from build123d import *

# Parameters (mm, degrees)
SKETCH1_W             = 25.4
SKETCH1_H             = 25.4
SKETCH1_W_2           = 19.05
SKETCH1_H_2           = 19.05
BOSS_EXTRUDE1_DEPTH   = 279.4
SKETCH3_W             = 2.4892
SKETCH3_H             = 25.4
SKETCH3_AT_POINT_2_W  = 2.4892
SKETCH3_AT_POINT_2_H  = 25.4
LPATTERN1_START       = -12.7
LPATTERN1_OUTLINE_R   = 2.4892
LPATTERN1_DEPTH       = 25.4
LPATTERN1_2_OUTLINE_R = 2.4892
LPATTERN1_2_DEPTH     = 25.4


# Read off the part's stored shape, not the designer's step: LPattern1
with BuildPart() as part:
    # Sketch1 → Boss-Extrude1 (new, symmetric)
    with BuildSketch(Plane(origin=(0, 0, 0), x_dir=(0, 0, -1), z_dir=(1, 0, 0))):
        Rectangle(SKETCH1_W, SKETCH1_H)
        Rectangle(SKETCH1_W_2, SKETCH1_H_2, mode=Mode.SUBTRACT)
    extrude(amount=BOSS_EXTRUDE1_DEPTH, both=True)

    # Sketch3 → #9 (0.196) Diameter Hole1 (revolve, cut)
    with BuildSketch(Plane(origin=(266.7, 12.7, 0), x_dir=(0, 0, 1), z_dir=(1, 0, 0))):
        with Locations((1.2446, 12.7)):
            Rectangle(SKETCH3_W, SKETCH3_H)
    revolve(axis=Axis((266.7, 19.05, 0), (0, -1, 0)), mode=Mode.SUBTRACT)

    # Sketch3 at point 2 (carried to point 2, square into its face) → #9 (0.196) Diameter Hole1 at 2 (revolve, cut)
    with BuildSketch(Plane(origin=(266.7, 0, 12.7), x_dir=(0, -1, 0), z_dir=(1, 0, 0))):
        with Locations((1.2446, 12.7)):
            Rectangle(SKETCH3_AT_POINT_2_W, SKETCH3_AT_POINT_2_H)
    revolve(axis=Axis((266.7, 0, 19.05), (0, 0, -1)), mode=Mode.SUBTRACT)

    # LPattern1 outline → LPattern1 (cut)
    with BuildSketch(Plane.XY.offset(LPATTERN1_START)):
        with Locations((241.3, 0)):
            Circle(LPATTERN1_OUTLINE_R)
        with Locations((215.9, 0)):
            Circle(LPATTERN1_OUTLINE_R)
        with Locations((190.5, 0)):
            Circle(LPATTERN1_OUTLINE_R)
        with Locations((165.1, 0)):
            Circle(LPATTERN1_OUTLINE_R)
        with Locations((139.7, 0)):
            Circle(LPATTERN1_OUTLINE_R)
        with Locations((114.3, 0)):
            Circle(LPATTERN1_OUTLINE_R)
        with Locations((88.9, 0)):
            Circle(LPATTERN1_OUTLINE_R)
        with Locations((63.5, 0)):
            Circle(LPATTERN1_OUTLINE_R)
        with Locations((38.1, 0)):
            Circle(LPATTERN1_OUTLINE_R)
        with Locations((12.7, 0)):
            Circle(LPATTERN1_OUTLINE_R)
        with Locations((-12.7, 0)):
            Circle(LPATTERN1_OUTLINE_R)
        with Locations((-38.1, 0)):
            Circle(LPATTERN1_OUTLINE_R)
        with Locations((-63.5, 0)):
            Circle(LPATTERN1_OUTLINE_R)
        with Locations((-88.9, 0)):
            Circle(LPATTERN1_OUTLINE_R)
        with Locations((-114.3, 0)):
            Circle(LPATTERN1_OUTLINE_R)
        with Locations((-139.7, 0)):
            Circle(LPATTERN1_OUTLINE_R)
        with Locations((-165.1, 0)):
            Circle(LPATTERN1_OUTLINE_R)
        with Locations((-190.5, 0)):
            Circle(LPATTERN1_OUTLINE_R)
        with Locations((-215.9, 0)):
            Circle(LPATTERN1_OUTLINE_R)
        with Locations((-241.3, 0)):
            Circle(LPATTERN1_OUTLINE_R)
        with Locations((-266.7, 0)):
            Circle(LPATTERN1_OUTLINE_R)
    extrude(amount=LPATTERN1_DEPTH, mode=Mode.SUBTRACT)

    # LPattern1 2 outline → LPattern1 2 (cut)
    with BuildSketch(Plane(origin=(0, 0, 0), x_dir=(1, 0, 0), z_dir=(0, 1, 0)).offset(LPATTERN1_START)):
        with Locations((241.3, 0)):
            Circle(LPATTERN1_2_OUTLINE_R)
        with Locations((215.9, 0)):
            Circle(LPATTERN1_2_OUTLINE_R)
        with Locations((190.5, 0)):
            Circle(LPATTERN1_2_OUTLINE_R)
        with Locations((165.1, 0)):
            Circle(LPATTERN1_2_OUTLINE_R)
        with Locations((139.7, 0)):
            Circle(LPATTERN1_2_OUTLINE_R)
        with Locations((114.3, 0)):
            Circle(LPATTERN1_2_OUTLINE_R)
        with Locations((88.9, 0)):
            Circle(LPATTERN1_2_OUTLINE_R)
        with Locations((63.5, 0)):
            Circle(LPATTERN1_2_OUTLINE_R)
        with Locations((38.1, 0)):
            Circle(LPATTERN1_2_OUTLINE_R)
        with Locations((12.7, 0)):
            Circle(LPATTERN1_2_OUTLINE_R)
        with Locations((-12.7, 0)):
            Circle(LPATTERN1_2_OUTLINE_R)
        with Locations((-38.1, 0)):
            Circle(LPATTERN1_2_OUTLINE_R)
        with Locations((-63.5, 0)):
            Circle(LPATTERN1_2_OUTLINE_R)
        with Locations((-88.9, 0)):
            Circle(LPATTERN1_2_OUTLINE_R)
        with Locations((-114.3, 0)):
            Circle(LPATTERN1_2_OUTLINE_R)
        with Locations((-139.7, 0)):
            Circle(LPATTERN1_2_OUTLINE_R)
        with Locations((-165.1, 0)):
            Circle(LPATTERN1_2_OUTLINE_R)
        with Locations((-190.5, 0)):
            Circle(LPATTERN1_2_OUTLINE_R)
        with Locations((-215.9, 0)):
            Circle(LPATTERN1_2_OUTLINE_R)
        with Locations((-241.3, 0)):
            Circle(LPATTERN1_2_OUTLINE_R)
        with Locations((-266.7, 0)):
            Circle(LPATTERN1_2_OUTLINE_R)
    extrude(amount=LPATTERN1_2_DEPTH, mode=Mode.SUBTRACT)


solid = part.part
For this review, take the finished solid that the model builds, in its own axes (mm). A direction names the side the tool comes from. Round coordinates to 2 decimals unless told otherwise and drop trailing zeros. Order: outer loops, then holes, each group sorted by start corner. A loop starts at its lowest first (then second) coordinate and runs counter-clockwise, first axis right, second up. Notation, with made-up numbers: M -29,86 L -1,86 A23 cw -1,105 Z; hole C -19,39 d6. An arc over 180 degrees is marked long. Write each question's results on one line, items separated by ' | '. Start each with the question number.
1. Add section A-A (x = 231). State the section outline as (y, z) points (3 decimals).
2. Draft analysis for pull direction Y (two halves, no side actions). For faces 3 (the face through (4, -12.7, 0)), 4 (the face through (-279.4, 0, -11)), 5 (the face through (4, 0, -9.525)), state which applies: pulls with the +Y half, pulls with the -Y half, needs draft (parallel to the pull), parting line crosses it, or undercut.
3. Tool access review of faces 1 (the face through (4, -9.525, 0)), 2 (the face through (4, 12.7, 0)): name each direction out of +Z, -Z, +X, -X, +Y, -Y from which nothing blocks a thin tool from reaching the whole face with its end or side.
4. To check wall thickness, follow L1, parallel to Z at x = -134, y = 7.75 (3 decimals); L2, parallel to Y at x = -38.1, z = -11.35. State the ranges of each line that lie inside material, in increasing order. Write a range as [from, to].
5. Clearance check with a flat-ended pin moving along its axis: pin 1 Ø8 at (x, y) = (190.5, 0) entering from -Z. State where the tip first meets the part, or that it passes through.
Output values:
1) outline: M -12.7,-12.7 L 12.7,-12.7 L 12.7,12.7 L -12.7,12.7 Z; hole M -9.525,-9.525 L 9.525,-9.525 L 9.525,9.525 L -9.525,9.525 Z
2) face 3: pulls with the -Y half | face 4: needs draft | face 5: undercut
3) face 1: +X, -X | face 2: +Z, -Z, +X, -X, +Y
4) L1: [-12.7, -9.525], [9.525, 12.7] | L2: [-12.7, -2.49], [2.49, 12.7]
5) pin 1: z = -12.7
